Build history of the part. All positions in model axes, mm. Face numbers are marked on the shaded views. A direction names the side the tool comes from. Give positions to 0.01 mm unless a question says otherwise; leave off trailing zeros. Write each loop counter-clockwise with the first axis right and the second up, starting at its lowest first coordinate (ties: lowest second). Pieces come first, ordered by that corner, then holes.
from build123d import *

# Parameters (mm, degrees)
CASE_40P7X19P7_START                 = -30
CASE_40P7X19P7_PROFILE_W             = 40.7
CASE_40P7X19P7_PROFILE_H             = 19.7
CASE_40P7X19P7_DEPTH                 = 37
MOUNTING_FLANGE_NOMINAL_START        = -3
MOUNTING_FLANGE_NOMINAL_PROFILE_W    = 53.7
MOUNTING_FLANGE_NOMINAL_PROFILE_H    = 19.7
MOUNTING_FLANGE_NOMINAL_DEPTH        = 3
OUTPUT_ENVELOPE_NOT_SPLINE_START     = 7
OUTPUT_ENVELOPE_NOT_SPLINE_PROFILE_R = 3
OUTPUT_ENVELOPE_NOT_SPLINE_DEPTH     = 5.9
TAB_HOLES_NOMINAL_START              = -50
TAB_HOLES_NOMINAL_PROFILE_R          = 1.75
TAB_HOLES_NOMINAL_DEPTH              = 99.794082633


with BuildPart() as part:
    # Case_40p7x19p7_profile → Case_40p7x19p7 (new body)
    with BuildSketch(Plane.XY.offset(CASE_40P7X19P7_START)):
        with Locations((10.35, 0)):
            Rectangle(CASE_40P7X19P7_PROFILE_W, CASE_40P7X19P7_PROFILE_H)
    extrude(amount=CASE_40P7X19P7_DEPTH)

    # Mounting_flange_nominal_profile → Mounting_flange_nominal (add)
    with BuildSketch(Plane.XY.offset(MOUNTING_FLANGE_NOMINAL_START)):
        with Locations((10.35, 0)):
            Rectangle(MOUNTING_FLANGE_NOMINAL_PROFILE_W, MOUNTING_FLANGE_NOMINAL_PROFILE_H)
    extrude(amount=MOUNTING_FLANGE_NOMINAL_DEPTH)

    # Output_envelope_not_spline_profile → Output_envelope_not_spline (add)
    with BuildSketch(Plane.XY.offset(OUTPUT_ENVELOPE_NOT_SPLINE_START)):
        Circle(OUTPUT_ENVELOPE_NOT_SPLINE_PROFILE_R)
    extrude(amount=OUTPUT_ENVELOPE_NOT_SPLINE_DEPTH)

    # Tab_holes_nominal_profile → Tab_holes_nominal (cut, through all)
    with BuildSketch(Plane.XY.offset(TAB_HOLES_NOMINAL_START)):
        with Locations(Location((-13, 5, 0), (0, 0, 180))):
            Circle(TAB_HOLES_NOMINAL_PROFILE_R)
        with Locations(Location((-13, -5, 0), (0, 0, 180))):
            Circle(TAB_HOLES_NOMINAL_PROFILE_R)
        with Locations(Location((34, 5, 0), (0, 0, 180))):
            Circle(TAB_HOLES_NOMINAL_PROFILE_R)
        with Locations(Location((34, -5, 0), (0, 0, 180))):
            Circle(TAB_HOLES_NOMINAL_PROFILE_R)
    extrude(amount=TAB_HOLES_NOMINAL_DEPTH, mode=Mode.SUBTRACT)


solid = part.part
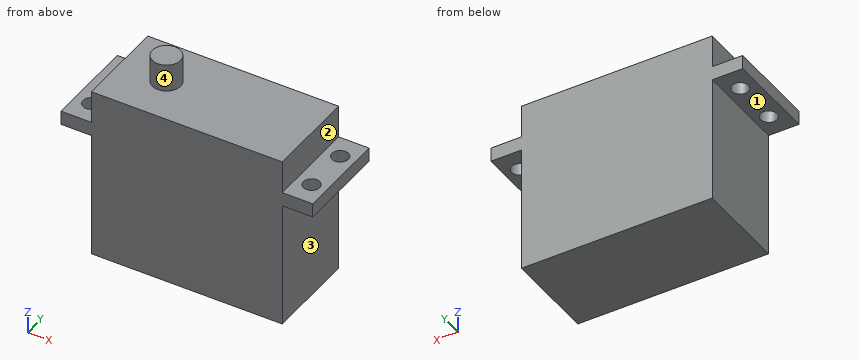
1. Saw through at D-D on z = -24. Give the cut face in (x, y).
2. Saw through at B-B on y = 5. Give the cut face in (x, z), plus the area to 3 significant figures.
3. Drop flat-ended pins along their axis: pin 1 (5.5 mm diameter, centred on x = 34, y = 5, fed in from +Z); pin 2 (5.5 mm diameter, centred on y = 0, z = 3.5, fed in from +X); pin 3 (1 mm diameter, centred on x = 16.5, y = -1.5, fed in from +Z). Give the stop position or say it passes through.
4. 3-axis set-ups, long thin cutter, end or side, ignore diameter. For the marked faces 1, 2, 3 and 4: which of +Z, -Z, +X, -X, +Y, -Y reach the whole face in a straight line?
5. Saw through at C-C on y = 0. Give the cut face in (x, z).
6. Saw through at A-A on x = 34. Give the cut face in (y, z), plus the area to 3 significant figures.
7. Drill centre lines: line 1 along Y through (x, z) = (34, -1.65); line 2 along Z through (x, y) = (9, 6.5); line 3 along Z through (x, y) = (31, -0.5). Where is each one in solid material? Low to high.
Outcome:
1. outline: (-10, -9.85) - (30.7, -9.85) - (30.7, 9.85) - (-10, 9.85) - close
2. outline: (-16.5, -3) - (-14.75, -3) - (-14.75, 0) - (-16.5, 0) - close; (-11.25, -3) - (-10, -3) - (-10, -30) - (30.7, -30) - (30.7, -3) - (32.25, -3) - (32.25, 0) - (30.7, 0) - (30.7, 7) - (-10, 7) - (-10, 0) - (-11.25, 0) - close; (35.75, -3) - (37.2, -3) - (37.2, 0) - (35.75, 0) - close
2. area: 1,520 mm2
3. pin 1: stops at z = 0
3. pin 2: stops at x = 30.7
3. pin 3: stops at z = 7
4. face 1: -Z, -X, +Y, -Y
4. face 2: +Z, +X, +Y, -Y
4. face 3: -Z, +X, +Y, -Y
4. face 4: +Z
5. outline: (-16.5, -3) - (-10, -3) - (-10, -30) - (30.7, -30) - (30.7, -3) - (37.2, -3) - (37.2, 0) - (30.7, 0) - (30.7, 7) - (3, 7) - (3, 12.9) - (-3, 12.9) - (-3, 7) - (-10, 7) - (-10, 0) - (-16.5, 0) - close
6. outline: (-9.85, -3) - (-6.75, -3) - (-6.75, 0) - (-9.85, 0) - close; (-3.25, -3) - (3.25, -3) - (3.25, 0) - (-3.25, 0) - close; (6.75, -3) - (9.85, -3) - (9.85, 0) - (6.75, 0) - close
6. area: 38.1 mm2
7. line 1: y = -9.85 to -6.75, -3.25 to 3.25, 6.75 to 9.85
7. line 2: z = -30 to 7
7. line 3: z = -3 to 0
